CAD build for the part. Positions are in the model's coordinates, mm. Face numbers are marked on the shaded views. Round coordinates to 2 decimals unless told otherwise and drop trailing zeros. Loops run counter-clockwise (first coordinate to the right, second up) from the corner with the lowest first, then second, coordinate; pieces in that order, holes last.
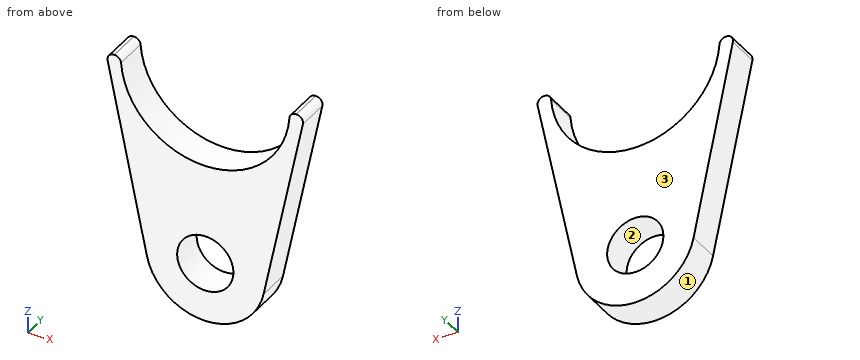
from build123d import *

# Parameters (mm, degrees)
F1_DEPTH = 5
F3_D     = 8.5
F4_R     = 1


with BuildPart() as f1:
    # F0 (on Front) → F1 (new body)
    with BuildSketch(Plane.XZ):
        with BuildLine():
            Line((-15, 0), (-8.812388, -29.828065))
            ThreePointArc((-8.812388, -29.828065), (0, -37), (8.812388, -29.828065))
            Line((8.812388, -29.828065), (15, 0))
            Line((15, 0), (12.75, 0))
            ThreePointArc((12.75, 0), (0, -12.75), (-12.75, 0))
            Line((-12.75, 0), (-15, 0))
        make_face()
    extrude(amount=F1_DEPTH)

    # F3 (through all)
    with Locations(Plane.XZ.offset(5)):
        with Locations((0, -28)):
            Hole(F3_D / 2)

    # F4
    f4_edges = [f1.edges().sort_by_distance(p)[0] for p in [
        (15, -2.5, 0),
        (-15, -2.5, 0),
        (-12.75, -2.5, 0),
        (12.75, -2.5, 0),
    ]]
    fillet(f4_edges, radius=F4_R)


solid = f1.part
Item 1: Mould opens along X. For the marked faces 1, 2 and 3 say: released by +X, released by -X, zero draft, split by the parting line, or undercut.
Verdict:
face 1: split by the parting line
face 2: undercut
face 3: zero draft
Item 2: Cut at B-B (y = -3.8). List the corners of the cut face in (x, z), plus the area to 3 significant figures.
Verdict:
outline: (-14.75, -1.2) - (-8.81, -29.83) arc R9 ccw to (8.81, -29.83) - (14.75, -1.2) arc R1 ccw to (13.77, 0) - (13.71, 0) arc R1 ccw to (12.72, -0.93) arc R12.75 cw to (-12.72, -0.93) arc R1 ccw to (-13.71, 0) - (-13.77, 0) arc R1 ccw to start; hole circle Ø8.5 at (0, -28)
area: 492 mm2
Item 3: Cut at C-C (z = -3.5). List the corners of the cut face in (x, y).
Verdict:
outline: (-14.27, -5) - (-12.26, -5) - (-12.26, 0) - (-14.27, 0) - close; (12.26, -5) - (14.27, -5) - (14.27, 0) - (12.26, 0) - close
Item 4: Cut at A-A (x = 0). List the corners of the cut face in (y, z).
Verdict:
outline: (-5, -37) - (0, -37) - (0, -32.25) - (-5, -32.25) - close; (-5, -23.75) - (0, -23.75) - (0, -12.75) - (-5, -12.75) - close
Item 5: Cut at D-D (x = -5.25). List the corners of the cut face in (y, z), plus the area to 3 significant figures.
Verdict:
outline: (-5, -35.31) - (0, -35.31) - (0, -11.62) - (-5, -11.62) - close
area: 118 mm2
Item 6: Flat gauge pins, fed straight in: P1, Ø8, axis at x = -2, z = -18, coming from the +Y side; P2, Ø3, axis at y = -1, z = -11, coming from the -X side. Where does each tip first touch, or does it go through?
Verdict:
P1: stops at y = 0
P2: stops at x = -13.03
Item 7: Wall check: L1, parallel to Z at x = 3.75, y = -4.4; L2, parallel to X at y = -4.45, z = -8; L3, parallel to Z at x = 1, y = -4.5. Give the ranges that are in metal, low to high.
Verdict:
L1: z = -36.18 to -30, -26 to -12.19
L2: x = -13.34 to -9.93, 9.93 to 13.34
L3: z = -36.94 to -32.13, -23.87 to -12.71
